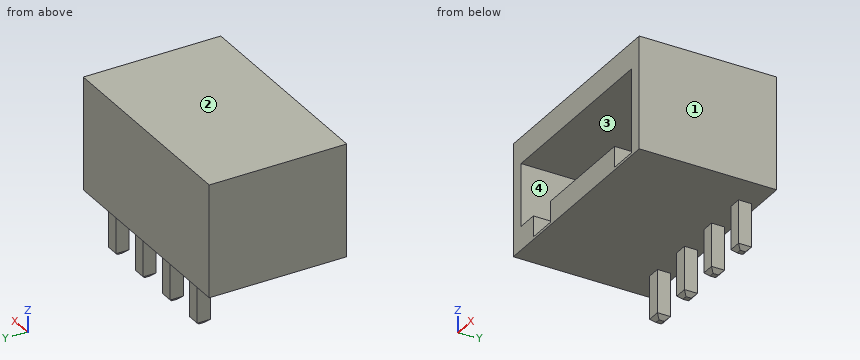
from build123d import *

# Parameters (mm, degrees)
SKETCH_1_W                         = 16.3
SKETCH_1_H                         = 10.5
EXTRUDE_1_DEPTH                    = 8.6
CUT_EXTRUDE_1_DEPTH                = 7
EXTRUDE_START                      = -5
SKETCH_3_W                         = 1
SKETCH_3_H                         = 1
EXTRUDE_2_DEPTH                    = 8.6
CHAMFER_1_SIZE                     = 0.3
PATTERN_LINEAR_1_COUNT             = 4
PATTERN_LINEAR_1_PITCH             = 3.5
CHAMFER_1_OF_PATTERN_LINEAR_1_SIZE = 0.3


with BuildPart() as part:
    # Эскиз1 → Бобышка-Вытянуть1 (new body)
    with BuildSketch(Plane.XY):
        Rectangle(SKETCH_1_W, SKETCH_1_H)
    extrude(amount=EXTRUDE_1_DEPTH)

    # Эскиз2 → Вырез-Вытянуть1 (cut)
    with BuildSketch(Plane.XZ.offset(5.25)):
        Polygon((-7.15, 6.6), (7.15, 6.6), (7.15, 0.2), (4.95, 0.2), (4.95, 1.8), (-3.35, 1.8), (-3.35, 0.2), (-5.55, 0.2), (-5.55, 1.8), (-7.15, 1.8), align=None)
    extrude(amount=-CUT_EXTRUDE_1_DEPTH, mode=Mode.SUBTRACT)

    # Эскиз3 → Бобышка-Вытянуть2 (add)
    with BuildSketch(Plane(origin=(0, 0, 0), x_dir=(-1, 0, 0), z_dir=(0, 0, -1)).offset(EXTRUDE_START)):
        with Locations((5.25, 4.25)):
            Rectangle(SKETCH_3_W, SKETCH_3_H)
    extrude_2 = extrude(amount=EXTRUDE_2_DEPTH)

    # Фаска1
    chamfer_1_edges = [part.edges().sort_by_distance(p)[0] for p in [
        (-4.75, 4.25, -3.6),
        (-5.25, 3.75, -3.6),
        (-5.75, 4.25, -3.6),
        (-5.25, 4.75, -3.6),
    ]]
    chamfer(chamfer_1_edges, length=CHAMFER_1_SIZE)

    # Линейный массив1: Бобышка-Вытянуть2 ×4
    with Locations(*[(i * PATTERN_LINEAR_1_PITCH, 0, 0) for i in range(1, PATTERN_LINEAR_1_COUNT)]):
        add(extrude_2)

    # Фаска1 of Линейный массив1
    chamfer_1_of_pattern_linear_1_edges = [part.edges().sort_by_distance(p)[0] for p in [
        (-1.25, 4.25, -3.6),
        (-1.75, 3.75, -3.6),
        (-2.25, 4.25, -3.6),
        (-1.75, 4.75, -3.6),
        (2.25, 4.25, -3.6),
        (1.75, 3.75, -3.6),
        (1.25, 4.25, -3.6),
        (1.75, 4.75, -3.6),
        (5.75, 4.25, -3.6),
        (5.25, 3.75, -3.6),
        (4.75, 4.25, -3.6),
        (5.25, 4.75, -3.6),
    ]]
    chamfer(chamfer_1_of_pattern_linear_1_edges, length=CHAMFER_1_OF_PATTERN_LINEAR_1_SIZE)


solid = part.part
Can you work these out from the model? Positions are in its coordinate system, mm. Face numbers are marked on the shaded views. Give positions to 0.01 mm unless a question says otherwise; leave off trailing zeros. Loops run counter-clockwise (first coordinate to the right, second up) from the corner with the lowest first, then second, coordinate; pieces in that order, holes last. Notation, with made-up numbers: (-40, -7.5) -> (19, -7.5) arc R14 cw to (19, 13.5) -> close; hole circle Ø9 at (-29.5, 20.25). An arc over 180 degrees is marked (long way). Write item = value, one per line.
1) I need wall thicknesses on L1, parallel to X at y = -4, z = 1.5; L2, parallel to X at y = 4.25, z = -0.25; L3, parallel to Z at x = 1, y = 0. Which ranges of each line are inside material? Lowest first, please. Write a range as from..to.
Check result:
L1 = -8.15..-5.55, -3.35..4.95, 7.15..8.15
L2 = -5.75..-4.75, -2.25..-1.25, 1.25..2.25, 4.75..5.75
L3 = 0..1.8, 6.6..8.6
2) Suppose I cut it at B-B on y = 1. Write out the boundary of the cut face in (x, z), then the cut area to 3 significant figures.
Check result:
outline = (-8.15, 0) -> (8.15, 0) -> (8.15, 8.6) -> (-8.15, 8.6) -> close; hole (-7.15, 1.8) -> (-5.55, 1.8) -> (-5.55, 0.2) -> (-3.35, 0.2) -> (-3.35, 1.8) -> (4.95, 1.8) -> (4.95, 0.2) -> (7.15, 0.2) -> (7.15, 6.6) -> (-7.15, 6.6) -> close
area = 64.5 mm2
3) Thinking about a two-plate mould opening in Z: for the marked faces 1, 2, 3 and 4, which applies, released by +Z, released by -Z, zero draft, split by the parting line, or undercut?
Check result:
face_1 = zero draft
face_2 = released by +Z
face_3 = undercut
face_4 = undercut
4) Suppose I cut it at C-C on x = 0.75. Write out the boundary of the cut face in (y, z), then the cut area to 3 significant figures.
Check result:
outline = (-5.25, 0) -> (5.25, 0) -> (5.25, 8.6) -> (-5.25, 8.6) -> (-5.25, 6.6) -> (1.75, 6.6) -> (1.75, 1.8) -> (-5.25, 1.8) -> close
area = 56.7 mm2
5) Will these pins go through, and if not, where does the flat tip stop? pin 1 (1.1 mm diameter, centred on x = -1.5, z = -1.5, fed in from +Y); pin 2 (0.8 mm diameter, centred on x = 5.5, z = -1.5, fed in from -Y); pin 3 (5 mm diameter, centred on x = 6.5, y = 1, fed in from -Z); pin 4 (5 mm diameter, centred on x = 2.5, z = 3.5, fed in from -Y).
Check result:
pin_1 = 4.75
pin_2 = 3.75
pin_3 = 0
pin_4 = -5.25
6) Suppose I cut it at A-A on z = -0.25. Write out the boundary of the cut face in (x, y).
Check result:
outline = (-5.75, 3.75) -> (-4.75, 3.75) -> (-4.75, 4.75) -> (-5.75, 4.75) -> close; (-2.25, 3.75) -> (-1.25, 3.75) -> (-1.25, 4.75) -> (-2.25, 4.75) -> close; (1.25, 3.75) -> (2.25, 3.75) -> (2.25, 4.75) -> (1.25, 4.75) -> close; (4.75, 3.75) -> (5.75, 3.75) -> (5.75, 4.75) -> (4.75, 4.75) -> close
7) Suppose I cut it at D-D on z = 6. Write out the boundary of the cut face in (x, y), then the cut area to 4 significant figures.
Check result:
outline = (-8.15, -5.25) -> (-7.15, -5.25) -> (-7.15, 1.75) -> (7.15, 1.75) -> (7.15, -5.25) -> (8.15, -5.25) -> (8.15, 5.25) -> (-8.15, 5.25) -> close
area = 71.05 mm2
